Could you check a few things on this model? Use its own coordinates, in mm. Round coordinates to 2 decimals unless told otherwise and drop trailing zeros. Loops run counter-clockwise (first coordinate to the right, second up) from the corner with the lowest first, then second, coordinate; pieces in that order, holes last. Notation, with made-up numbers: M 14,81.5 L 45,81.5 A20 cw 45,107.5 Z; hole C -14.5,-24.5 d3. An arc over 180 degrees is marked long. One line per item, written item: value. Start each with the question number.
Q1. Imagine slicing it at A-A (y = 0). Please give me the cut outline in (x, z).
Q2. Please list where these lines run through material, in increasing order: line 1 along X through (y, z) = (-1.5, -0.55); line 2 along X through (y, z) = (-0.5, -0.45); line 3 along Y through (x, z) = (0, -1).
Q3. I'm going to push a flat-ended pin straight in: pin 1 Ø15 at (x, y) = (425, 0) entering from +Z. Where does the tip first touch, or does it pass through?
from build123d import *

# Parameters (mm, degrees)
PLAT_W                          = 30
PLAT_H                          = 5
EL_MENT_M_CANO_SOUD_1_DEPTH     = 1820
DIAM_TRE_DU_PER_AGE_13_0_13_1_D = 13
R_P_TITION_LIN_AIRE2_COUNT      = 5
R_P_TITION_LIN_AIRE2_PITCH      = 425


with BuildPart() as part:
    # plat → Elément mécano-soudé1 (new body)
    with BuildSketch(Plane.YZ.offset(-910)):
        Rectangle(PLAT_W, PLAT_H)
    extrude(amount=EL_MENT_M_CANO_SOUD_1_DEPTH)

    # Diamètre du perçage Ø13.0 (13)1 (through all)
    with Locations(Plane(origin=(0, 0, -2.5), x_dir=(-1, 0, 0), z_dir=(0, 0, -1))):
        with Locations((850, 0)):
            diam_tre_du_per_age_13_0_13_1 = Hole(DIAM_TRE_DU_PER_AGE_13_0_13_1_D / 2)

    # Répétition linéaire2: Diamètre du perçage Ø13.0 (13)1 ×5
    with Locations(*[(i * R_P_TITION_LIN_AIRE2_PITCH, 0, 0) for i in range(1, R_P_TITION_LIN_AIRE2_COUNT)]):
        add(diam_tre_du_per_age_13_0_13_1, mode=Mode.SUBTRACT)


solid = part.part
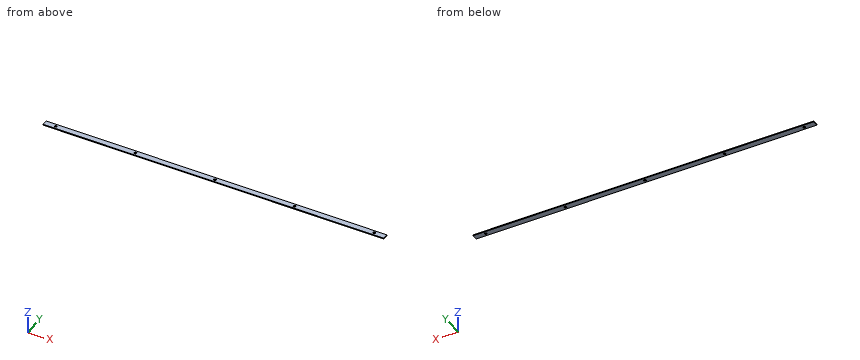
Report:
1. outline: M -910,-2.5 L -856.5,-2.5 L -856.5,2.5 L -910,2.5 Z; M -843.5,-2.5 L -431.5,-2.5 L -431.5,2.5 L -843.5,2.5 Z; M -418.5,-2.5 L -6.5,-2.5 L -6.5,2.5 L -418.5,2.5 Z; M 6.5,-2.5 L 418.5,-2.5 L 418.5,2.5 L 6.5,2.5 Z; M 431.5,-2.5 L 843.5,-2.5 L 843.5,2.5 L 431.5,2.5 Z; M 856.5,-2.5 L 910,-2.5 L 910,2.5 L 856.5,2.5 Z
2. line 1: x = -910 to -856.32, -843.68 to -431.32, -418.68 to -6.32, 6.32 to 418.68, 431.32 to 843.68, 856.32 to 910
2. line 2: x = -910 to -856.48, -843.52 to -431.48, -418.52 to -6.48, 6.48 to 418.52, 431.48 to 843.52, 856.48 to 910
2. line 3: y = -15 to -6.5, 6.5 to 15
3. pin 1: stops at z = 2.5
